CAD build for the part. Positions are in the model's coordinates, mm. A direction names the side the tool comes from. Give positions to 0.01 mm unless a question says otherwise; leave off trailing zeros. Loops run counter-clockwise (first coordinate to the right, second up) from the corner with the lowest first, then second, coordinate; pieces in that order, holes last.
Autodesk Inventor part; units mm, degrees
ref_plane "YZ Plane" through (0, 0, 0) normal (1, 0, 0) x (0, 1, 0)
ref_plane "XZ Plane" through (0, 0, 0) normal (0, 1, 0) x (-1, 0, 0)
ref_plane "XY Plane" through (0, 0, 0) normal (0, 0, 1) x (1, 0, 0)
sketch "Sketch3" plane through (0, 0, 0) normal (1, 0, 0) x (0, 1, 0)
  circle A0 centre (0, 0) radius 15.875 construction
  circle A1 centre (0, 0) radius 14.6304
  dimension "d8" = 31.75
  dimension "d9" = 1.2446
extrude "Extrusion3" add sketch "Sketch3" along normal blind 12.7
sketch "Sketch4" plane through (12.7, 0, 0) normal (1, 0, 0) x (0, 0, -1)
  circle A0 centre (0, 0) radius 4.7625
  dimension "d12" = 9.525
extrude "Extrusion4" add sketch "Sketch4" along normal blind 41.275
sketch "Sketch5" plane through (53.975, 0, 0) normal (1, 0, 0) x (0, 0, -1)
  circle A0 centre (0, 0) radius 2.4892
  dimension "d15" = 4.9784
extrude "Extrusion5" cut sketch "Sketch5" against normal blind 25.4
sketch "Sketch6" plane through (0, 0, 0) normal (-1, 0, 0) x (0, 0, 1)
  circle A0 centre (0, 0) radius 9.525
  dimension "d18" = 19.05
extrude "Extrusion6" cut sketch "Sketch6" against normal blind 9.525
properties part number "Long roller plug 3"
1. Probe line 1 along Y through (x, z) = (48, 0); line 2 along X through (y, z) = (9.75, -7); line 3 along X through (y, z) = (2.25, 8.5) (3 decimals). List the from-to ranges inside material, lowest first.
Responses:
line 1: y = -4.76 to -2.49, 2.49 to 4.76
line 2: x = 0 to 12.7
line 3: x = 9.525 to 12.7
2. Saw through at C-C, the plane x = 22.5. List the corners of the cut face in (y, z) (1 decimal), and give its area (3 significant figures).
Responses:
outline: circle Ø9.5 at (0, 0)
area: 71.3 mm2
3. Tool access for faces 4 (the face through (4.696, -5.796, -7.559)), 5 (the face through (53.975, -2, -2)), 6 (the face through (28.575, 0, 0)): list every direction of +Z, -Z, +X, -X, +Y, -Y with a clear straight run to the whole face (end or side of a thin tool).
Responses:
face 4: -X
face 5: +Z, -Z, +X, +Y, -Y
face 6: +X
4. Drop flat-ended pins along their axis: pin 1 (5 mm diameter, centred on x = 45.5, y = -6, fed in from -Z); pin 2 (6 mm diameter, centred on x = 26, y = -5, fed in from -Z); pin 3 (5.5 mm diameter, centred on y = -1.5, z = 4, fed in from -X) (3 decimals). Give the stop position or say it passes through.
Responses:
pin 1: stops at z = -3.23
pin 2: stops at z = -4.32
pin 3: stops at x = 9.525
5. Saw through at D-D, the plane y = -3.5. List the corners of the cut face in (x, z) (3 decimals).
Responses:
outline: (0, -14.206) - (12.7, -14.206) - (12.7, -3.23) - (53.975, -3.23) - (53.975, 3.23) - (12.7, 3.23) - (12.7, 14.206) - (0, 14.206) - (0, 8.859) - (9.525, 8.859) - (9.525, -8.859) - (0, -8.859) - close
6. Saw through at A-A, the plane y = 0. List the corners of the cut face in (x, z) (1 decimal), and give its area (3 significant figures).
Responses:
outline: (0, -14.6) - (12.7, -14.6) - (12.7, -4.8) - (54, -4.8) - (54, -2.5) - (28.6, -2.5) - (28.6, 2.5) - (54, 2.5) - (54, 4.8) - (12.7, 4.8) - (12.7, 14.6) - (0, 14.6) - (0, 9.5) - (9.5, 9.5) - (9.5, -9.5) - (0, -9.5) - close
area: 457 mm2
7. Pull direction Y, two halves, no side cores. Call faces 1 (the face through (12.7, -3.5, 3.5)), 2 (the face through (33.05, 2.9, 3.78)), 3 (the face through (41.453, 0.748, -2.374)): released by +Y, released by -Y, zero draft, split by the parting line, or undercut.
Responses:
face 1: zero draft
face 2: split by the parting line
face 3: undercut
